Model file for the job. Use its own axes, mm. Face numbers are marked on the shaded views. Coordinates: 2 decimals unless noted, no trailing zeros. Write each loop counter-clockwise with the first axis right and the second up, starting at its lowest first coordinate (ties: lowest second). Pieces come first, ordered by that corner, then holes.
Q1. Pin check, flat tips, straight feed: P1, Ø4, axis at x = -14.5, z = 6, coming from the +Y side; P2, Ø8, axis at y = 17.5, z = 19, coming from the -X side; P3, Ø10, axis at x = -9.5, z = -23, coming from the +Y side. Stop position of each tip, or through.
Q2. Pull direction Y, two halves, no side cores. Call the marked faces 1, 2 and 3: released by +Y, released by -Y, zero draft, split by the parting line, or undercut.
Q3. Drill centre lines: probe 1 along Z at (x, y) = (2.5, 2.5) (3 decimals); probe 2 along Y at (x, z) = (4, 0.5) (3 decimals); probe 3 along Y at (x, z) = (-8.5, 0.5) (3 decimals). Where is each one in solid material? Low to high.
Q4. Band-saw the part on C-C, the plane y = 21.5. Write the cut outline in (x, z) (3 decimals), plus the area to 3 significant figures.
Q5. Band-saw the part on B-B, the plane x = 8.5. Write the cut outline in (y, z) (3 decimals), plus the area to 3 significant figures.
Q6. Band-saw the part on A-A, the plane z = 8.5. Write the cut outline in (x, y) (3 decimals).
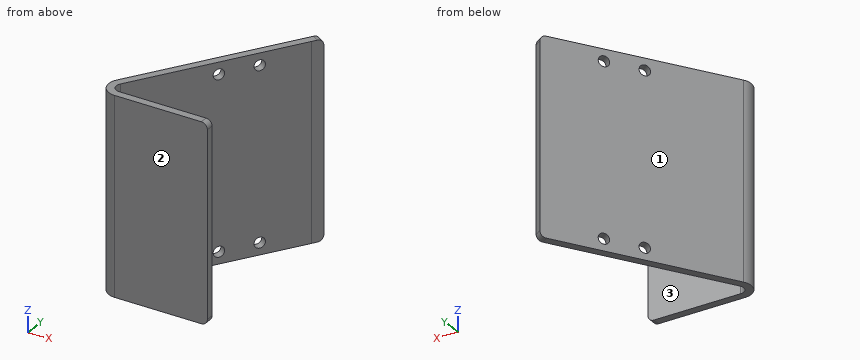
from build123d import *

# Parameters (mm, degrees)
BOSS_EXTRUDE1_DEPTH    = 41.275
CONVERT_SOLID1_START   = -41.275
CONVERT_SOLID1_DEPTH   = 82.55
CONVERT_SOLID1_2_DEPTH = 82.55
CUT_EXTRUDE1_REACH     = 64.782
SKETCH6_R              = 2.2479
FILLET1_R              = 2.54


# Read off the part's stored shape, not the designer's step: Convert-Solid1
with BuildPart() as part:
    # Sketch1 → Boss-Extrude1 (new, symmetric)
    with BuildSketch(Plane.XY):
        Polygon((25.4, -38.1), (-25.4, -38.1), (25.4, 38.1), align=None)
    extrude(amount=BOSS_EXTRUDE1_DEPTH, both=True)

    # Convert-Solid1 outline → Convert-Solid1 (cut)
    with BuildSketch(Plane.XY.offset(CONVERT_SOLID1_START)):
        with BuildLine():
            Line((25.4, -34.925), (25.4, 32.37618735))
            Line((25.4, 32.37618735), (-16.176676151, -29.988826877))
            ThreePointArc((-16.176676151, -29.988826877), (-16.334233318, -33.248148914), (-13.534916467, -34.925))
            Line((-13.534916467, -34.925), (25.4, -34.925))
        make_face()
        with BuildLine():
            ThreePointArc((-13.534916467, -38.1), (-19.133550169, -34.746297827), (-18.818435836, -28.227653754))
            Line((-18.818435836, -28.227653754), (-25.4, -38.1))
            Line((-25.4, -38.1), (-13.534916467, -38.1))
        make_face()
    extrude(amount=CONVERT_SOLID1_DEPTH, mode=Mode.SUBTRACT)

    # Convert-Solid1 2 outline → Convert-Solid1 2 (add)
    with BuildSketch(Plane.XY.offset(CONVERT_SOLID1_START)):
        Polygon((28.041759685, 36.338826877), (25.4, 38.1), (25.4, 32.37618735), align=None)
    extrude(amount=CONVERT_SOLID1_2_DEPTH)

    # Sketch6 → Cut-Extrude1 (cut, up to next)
    with BuildSketch(Plane(origin=(0, 0, 0), x_dir=(0, 0, 1), z_dir=(-0.8320502943378438, 0.554700196225229, 0)), mode=Mode.PRIVATE) as cut_extrude1_sk1:
        with Locations(Location((-36.2458, 20.701, 0), (0, 0, 270))):
            Circle(SKETCH6_R)
    cut_extrude1_tool1 = extrude(cut_extrude1_sk1.sketch, amount=-CUT_EXTRUDE1_REACH, mode=Mode.PRIVATE) & part.part
    # Sketch6 → Cut-Extrude1 (cut, up to next)
    with BuildSketch(Plane(origin=(0, 0, 0), x_dir=(0, 0, 1), z_dir=(-0.8320502943378438, 0.554700196225229, 0)), mode=Mode.PRIVATE) as cut_extrude1_sk2:
        with Locations(Location((36.2458, 20.701, 0), (0, 0, 270))):
            Circle(SKETCH6_R)
    cut_extrude1_tool2 = extrude(cut_extrude1_sk2.sketch, amount=-CUT_EXTRUDE1_REACH, mode=Mode.PRIVATE) & part.part
    # Sketch6 → Cut-Extrude1 (cut, up to next)
    with BuildSketch(Plane(origin=(0, 0, 0), x_dir=(0, 0, 1), z_dir=(-0.8320502943378438, 0.554700196225229, 0)), mode=Mode.PRIVATE) as cut_extrude1_sk3:
        with Locations(Location((-36.2458, 4.699, 0), (0, 0, 270))):
            Circle(SKETCH6_R)
    cut_extrude1_tool3 = extrude(cut_extrude1_sk3.sketch, amount=-CUT_EXTRUDE1_REACH, mode=Mode.PRIVATE) & part.part
    # Sketch6 → Cut-Extrude1 (cut, up to next)
    with BuildSketch(Plane(origin=(0, 0, 0), x_dir=(0, 0, 1), z_dir=(-0.8320502943378438, 0.554700196225229, 0)), mode=Mode.PRIVATE) as cut_extrude1_sk4:
        with Locations(Location((36.2458, 4.699, 0), (0, 0, 270))):
            Circle(SKETCH6_R)
    cut_extrude1_tool4 = extrude(cut_extrude1_sk4.sketch, amount=-CUT_EXTRUDE1_REACH, mode=Mode.PRIVATE) & part.part
    add(cut_extrude1_tool1.solids().sort_by_distance((11.482849, 17.224273, -36.2458))[0], mode=Mode.SUBTRACT)
    add(cut_extrude1_tool2.solids().sort_by_distance((11.482849, 17.224273, 36.2458))[0], mode=Mode.SUBTRACT)
    add(cut_extrude1_tool3.solids().sort_by_distance((2.606536, 3.909804, -36.2458))[0], mode=Mode.SUBTRACT)
    add(cut_extrude1_tool4.solids().sort_by_distance((2.606536, 3.909804, 36.2458))[0], mode=Mode.SUBTRACT)

    # Fillet1
    fillet1_edges = [part.edges().sort_by_distance(p)[0] for p in [
        (26.720879842, 37.219413438, -41.275),
        (26.720879842, 37.219413438, 41.275),
        (25.4, -36.5125, 41.275),
        (25.4, -36.5125, -41.275),
    ]]
    fillet(fillet1_edges, radius=FILLET1_R)


solid = part.part
Answer sheet:
1. P1: stops at y = -18.75
1. P2: stops at x = 9
1. P3: stops at y = -6.75
2. face 1: released by +Y
2. face 2: released by -Y
2. face 3: undercut
3. probe 1: z = -41.275 to -38.126, -34.366 to 34.366, 38.126 to 41.275
3. probe 2: y = -38.1 to -34.925, 0.276 to 6
3. probe 3: y = -38.1 to -34.925, -18.474 to -12.75
4. outline: (14.333, -41.275) - (18.149, -41.275) - (18.149, 41.275) - (14.333, 41.275) - close
4. area: 315 mm2
5. outline: (-38.1, -41.275) - (-34.925, -41.275) - (-34.925, 41.275) - (-38.1, 41.275) - close; (7.026, -41.275) - (12.75, -41.275) - (12.75, 41.275) - (7.026, 41.275) - close
5. area: 735 mm2
6. outline: (-18.818, -28.228) arc R6.35 ccw to (-13.535, -38.1) - (25.4, -38.1) - (25.4, -34.925) - (-13.535, -34.925) arc R3.175 cw to (-16.177, -29.989) - (28.042, 36.339) - (25.4, 38.1) - close
